Here's the drawing with two shaded views (mm, measured from the low corner). I have some questions. A direction names the side the tool comes from. Give positions to 0.01 mm unless a question says otherwise; leave off trailing zeros. Loops run counter-clockwise (first coordinate to the right, second up) from the corner with the lowest first, then second, coordinate; pieces in that order, holes last. Notation, with made-up numbers: (55, -7.75) - (112, -7.75) arc R33 cw to (112, 21.25) - close; hole circle Ø7 at (-0.5, 54). An arc over 180 degrees is marked (long way). Use a Markdown table: item, result. Add a question column.
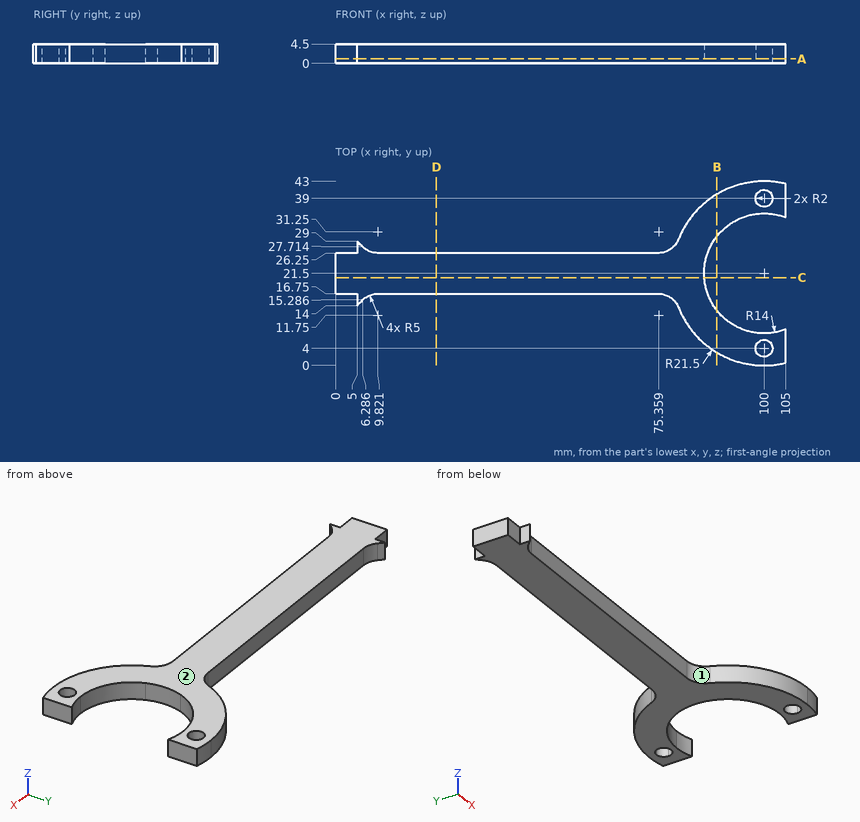
1. Suppose I cut it at D-D (x = 23.5). List the corners of the cut face in (y, z) for me.
2. Suppose I cut it at B-B (x = 89). List the corners of the cut face in (y, z) for me.
3. Please list where these lines run through material, in increasing order: line 1 along Y through (x, z) = (101, 2.4) (1 decimal); line 2 along Y through (x, z) = (51, 0.6); line 3 along Y through (x, z) = (99.5, 0.4) (1 decimal). Write a range as [from, to].
4. Suppose I cut it at A-A (z = 1). State how many separate pieces and enclosed holes the cut face has, and give its area (3 significant figures).
5. On a 3-axis mill with a long thin cutter (end or side, diameter ignored), from which of +Z, -Z, +X, -X, +Y, -Y can I reach the whole of each face in a straight line? I mean the marked faces 1 and 2. Say none if no direction works.
6. Will these pins go through, and if not, where does the flat tip stop? P1, Ø2, axis at x = 2, z = 2, coming from the -Y side; P2, Ø1, axis at y = 37.5, z = 3.5, coming from the -X side; P3, Ø1, axis at y = 15, z = 3.5, coming from the +X side (1 decimal).
7. Suppose I cut it at C-C (y = 20.5). List the corners of the cut face in (x, z) for me (1 decimal).
Results below:
| question | item | result |
|---|---|---|
| 1 | outline | (16.75, 0) - (26.25, 0) - (26.25, 4.5) - (16.75, 4.5) - close |
| 2 | outline | (3.03, 0) - (12.84, 0) - (12.84, 4.5) - (3.03, 4.5) - close; (30.16, 0) - (39.97, 0) - (39.97, 4.5) - (30.16, 4.5) - close |
| 3 | line 1 | [0, 2.3], [5.7, 7.5], [35.5, 37.3], [40.7, 43] |
| 3 | line 2 | [16.75, 26.25] |
| 3 | line 3 | [0, 2.1], [5.9, 7.5], [35.5, 37.1], [40.9, 43] |
| 4 | separate pieces | 1 |
| 4 | enclosed holes | 2 |
| 4 | area | 1,230 mm² |
| 5 | face 1 | +Z, -Z, -Y |
| 5 | face 2 | +Z, +X, -X, +Y, -Y |
| 6 | P1 | y = 16.75 |
| 6 | P2 | x = 85.1 |
| 6 | P3 | x = 87.9 |
| 7 | outline | (0, 0) - (86, 0) - (86, 4.5) - (0, 4.5) - close |
